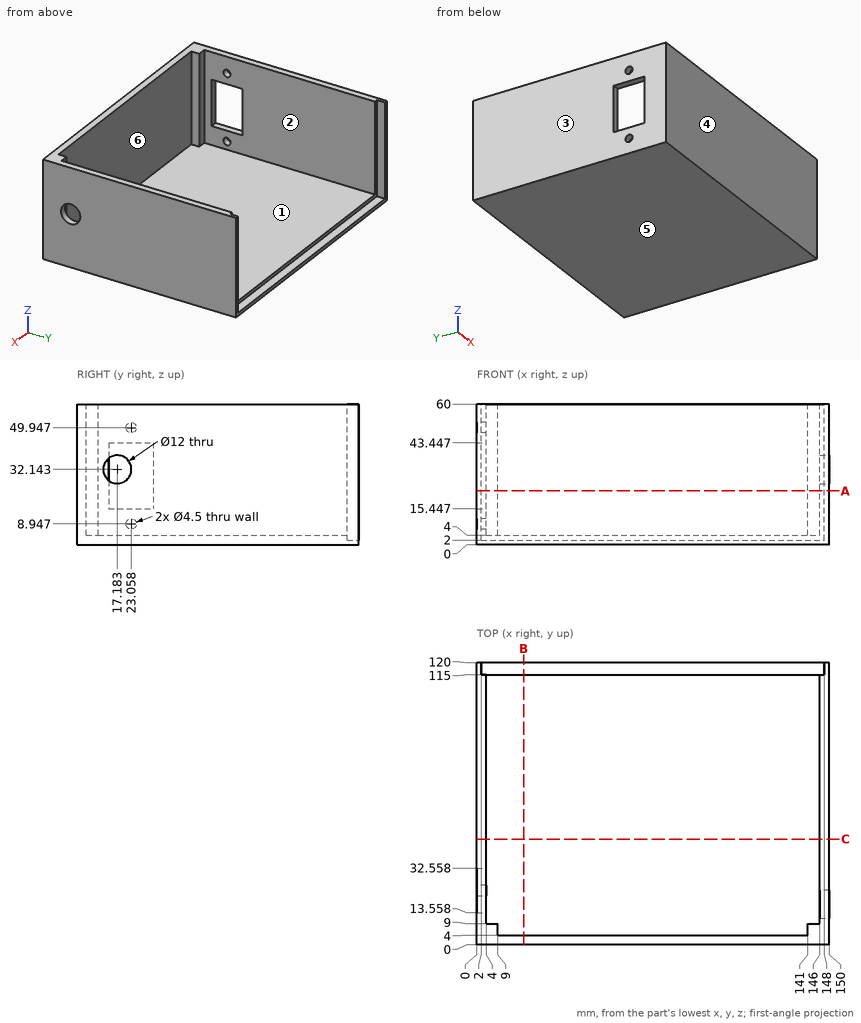
Source: three-view drawing plus pictorial views. Frame: mm from the lowest corner of the part. A direction names the side the tool comes from. Coordinates: 2 decimals unless noted, no trailing zeros. Loops run counter-clockwise (first coordinate to the right, second up) from the corner with the lowest first, then second, coordinate; pieces in that order, holes last. Notation, with made-up numbers: (55.5, 52.5) -> (109.5, 52.5) arc R26 ccw to (109.5, 83.5) -> close; hole circle Ø3 at (74.5, 18.5). An arc over 180 degrees is marked (long way). Answer in a Markdown table with one row per item. Add a question column.
Q1. Reachability of the marked faces 5 and 6 from +Z, -Z, +X, -X, +Y, -Y: full face, straight path, thin tool, end or side. Return the list, or none.
Q2. Section C-C on y = 45. Return the cut outline in (x, z).
Q3. Contact query for flat-ended pins moving along their axis: pin 1 Ø3.5 at (y, z) = (23.06, 8.95) entering from -X; pin 2 Ø1.5 at (x, z) = (5.5, 22.5) entering from +Y; pin 3 Ø8 at (x, z) = (94.5, 26) entering from +Y. Output: stop coordinate, or through.
Q4. Section A-A on z = 23. Return the cut outline in (x, y), and give its area (3 significant figures).
Q5. Pull-direction query (X, two-part tool) for the marked faces 1, 2, 3 and 4; classes: pulls with the +X half, pulls with the -X half, needs draft (parallel to the pull), parting line crosses it, or undercut.
Q6. Ray query, line 1 along X through (y, z) = (9.5, 6.5); line 2 along X through (y, z) = (8, 57); line 3 along Z through (x, y) = (11, 113). Return the intervals inside material, ascending.
Q7. Section B-B on x = 20. Return the cut outline in (y, z).
Computed values:
| question | item | result |
|---|---|---|
| 1 | face 5 | -Z, +X, -X, +Y, -Y |
| 1 | face 6 | +Z, +Y |
| 2 | outline | (0, 0) -> (150, 0) -> (150, 60) -> (146, 60) -> (146, 4) -> (4, 4) -> (4, 60) -> (0, 60) -> close |
| 3 | pin 1 | stops at x = 146 |
| 3 | pin 2 | stops at y = 9 |
| 3 | pin 3 | stops at y = 4 |
| 4 | outline | (0, 0) -> (150, 0) -> (150, 120) -> (148, 120) -> (148, 115) -> (146, 115) -> (146, 9) -> (141, 9) -> (141, 4) -> (9, 4) -> (9, 9) -> (4, 9) -> (4, 13.56) -> (0, 13.56) -> close; (0, 32.56) -> (4, 32.56) -> (4, 115) -> (2, 115) -> (2, 120) -> (0, 120) -> close |
| 4 | area | 1,480 mm^2 |
| 5 | face 1 | undercut |
| 5 | face 2 | undercut |
| 5 | face 3 | pulls with the -X half |
| 5 | face 4 | needs draft |
| 6 | line 1 | x = 0 to 4, 146 to 150 |
| 6 | line 2 | x = 0 to 9, 141 to 150 |
| 6 | line 3 | z = 0 to 4 |
| 7 | outline | (0, 0) -> (120, 0) -> (120, 2) -> (115, 2) -> (115, 4) -> (4, 4) -> (4, 60) -> (0, 60) -> close |
